For this review, take the finished solid that the model builds, in its own axes (mm). A direction names the side the tool comes from. Coordinates: 2 decimals unless noted, no trailing zeros. Loops run counter-clockwise (first coordinate to the right, second up) from the corner with the lowest first, then second, coordinate; pieces in that order, holes last. Notation, with made-up numbers: M 30,21 L 85,21 A31 cw 85,53 Z; hole C -7.5,-29 d6. An arc over 180 degrees is marked long. Use one line per item in the form item = value.
```python
from build123d import *

# Parameters (mm, degrees)
SKETCH1_W               = 32
SKETCH1_H               = 128
BOSS_EXTRUDE1_DEPTH     = 4
SKETCH4_R               = 1.25
CUT_EXTRUDE2_DEPTH      = 10
SKETCH5_R               = 1.25
CUT_EXTRUDE3_DEPTH      = 10
CUT_EXTRUDE4_DEPTH      = 1.65
LPATTERN3_COUNT         = 4
LPATTERN3_PITCH         = 32
CUT_EXTRUDE5_DEPTH      = 1.65
LPATTERN4_COUNT         = 4
LPATTERN4_PITCH         = 32
SKETCH8_W               = 24.3
SKETCH8_H               = 24.3
CUT_EXTRUDE6_DEPTH      = 10
BOSS_EXTRUDE2_DEPTH     = 4.5
SKETCH11_W              = 10.2
SKETCH11_H              = 71.7
CUT_EXTRUDE7_DEPTH      = 72.92530848
CUT_EXTRUDE8_DEPTH      = 3
SKETCH12_R              = 2.25
CUT_EXTRUDE9_DEPTH      = 3
MIRROR3_COPY_1_DEPTH    = 3
MIRROR3_COPY_2_SKETCH_R = 2.25
MIRROR3_COPY_2_DEPTH    = 3
SKETCH14_W              = 22
SKETCH14_H              = 3.85
CUT_EXTRUDE13_DEPTH     = 10


with BuildPart() as part:
    # Sketch1 → Boss-Extrude1 (new body)
    with BuildSketch(Plane(origin=(0, 0, 0), x_dir=(1, 0, 0), z_dir=(0, 1, 0))):
        Rectangle(SKETCH1_W, SKETCH1_H)
    extrude(amount=BOSS_EXTRUDE1_DEPTH)

    # Sketch4 → Cut-Extrude2 (cut)
    with BuildSketch(Plane.XZ):
        with Locations(Location((13.4, 61.4, 0), (0, 0, 270))):
            Circle(SKETCH4_R)
    cut_extrude2 = extrude(amount=-CUT_EXTRUDE2_DEPTH, mode=Mode.SUBTRACT)

    # Sketch5 → Cut-Extrude3 (cut)
    with BuildSketch(Plane.XZ):
        with Locations(Location((-13.4, -61.4, 0), (0, 0, 270))):
            Circle(SKETCH5_R)
    cut_extrude3 = extrude(amount=-CUT_EXTRUDE3_DEPTH, mode=Mode.SUBTRACT)

    # Sketch6 → Cut-Extrude4 (cut)
    with BuildSketch(Plane(origin=(0, 4, 0), x_dir=(1, 0, 0), z_dir=(0, 1, 0))):
        Polygon((-15.400518683, 62.555), (-13.4, 63.71), (-11.399481317, 62.555), (-11.399481317, 60.245), (-13.4, 59.09), (-15.400518683, 60.245), align=None)
    cut_extrude4 = extrude(amount=-CUT_EXTRUDE4_DEPTH, mode=Mode.SUBTRACT)

    # LPattern3: Cut-Extrude3, Cut-Extrude4 ×4
    with Locations(*[(0, 0, i * LPATTERN3_PITCH) for i in range(1, LPATTERN3_COUNT)]):
        add(cut_extrude3, mode=Mode.SUBTRACT)
        add(cut_extrude4, mode=Mode.SUBTRACT)

    # Sketch7 → Cut-Extrude5 (cut)
    with BuildSketch(Plane(origin=(0, 4, 0), x_dir=(1, 0, 0), z_dir=(0, 1, 0))):
        Polygon((13.4, -59.09), (11.399481317, -60.245), (11.399481317, -62.555), (13.4, -63.71), (15.400518683, -62.555), (15.400518683, -60.245), align=None)
    cut_extrude5 = extrude(amount=-CUT_EXTRUDE5_DEPTH, mode=Mode.SUBTRACT)

    # LPattern4: Cut-Extrude2, Cut-Extrude5 ×4
    with Locations(*[(0, 0, -i * LPATTERN4_PITCH) for i in range(1, LPATTERN4_COUNT)]):
        add(cut_extrude2, mode=Mode.SUBTRACT)
        add(cut_extrude5, mode=Mode.SUBTRACT)

    # Sketch8 → Cut-Extrude6 (cut)
    with BuildSketch(Plane.XZ):
        with Locations((0, 48)):
            Rectangle(SKETCH8_W, SKETCH8_H)
    cut_extrude6 = extrude(amount=-CUT_EXTRUDE6_DEPTH, mode=Mode.SUBTRACT)

    # Mirror1: Cut-Extrude6 across plane
    add(cut_extrude6.mirror(Plane.XY), mode=Mode.SUBTRACT)

    # Sketch9 → Boss-Extrude2 (add)
    with BuildSketch(Plane(origin=(0, 0, -64), x_dir=(-1, 0, 0), z_dir=(0, 0, -1))):
        Polygon((-16, 12), (-5, 12), (-5, 15), (5, 15), (5, 12), (16, 12), (16, -8), (5, -8), (5, -11), (-5, -11), (-5, -8), (-16, -8), align=None)
    boss_extrude2 = extrude(amount=BOSS_EXTRUDE2_DEPTH)

    # Sketch11 → Cut-Extrude7 (cut, through all)
    with BuildSketch(Plane.XZ):
        Rectangle(SKETCH11_W, SKETCH11_H)
    extrude(amount=-CUT_EXTRUDE7_DEPTH, mode=Mode.SUBTRACT)

    # Sketch10 → Cut-Extrude8 (cut)
    with BuildSketch(Plane.XY.offset(-64)):
        Polygon((-2.52, 13.864768035), (2.52, 13.864768035), (5.04, 9.5), (2.52, 5.135231965), (-2.52, 5.135231965), (-5.04, 9.5), align=None)
    cut_extrude8 = extrude(amount=-CUT_EXTRUDE8_DEPTH, mode=Mode.SUBTRACT)

    # Sketch12 → Cut-Extrude9 (cut)
    with BuildSketch(Plane.XY.offset(-67)):
        with Locations((0, 9.5)):
            Circle(SKETCH12_R)
    cut_extrude9 = extrude(amount=-CUT_EXTRUDE9_DEPTH, mode=Mode.SUBTRACT)

    # Mirror2: Cut-Extrude8, Cut-Extrude9 across plane
    add(cut_extrude8.mirror(Plane.ZX.offset(2)), mode=Mode.SUBTRACT)
    add(cut_extrude9.mirror(Plane.ZX.offset(2)), mode=Mode.SUBTRACT)

    # Mirror3: Boss-Extrude2, Cut-Extrude8, Cut-Extrude9 across plane
    add(boss_extrude2.mirror(Plane.XY))
    add(cut_extrude8.mirror(Plane.XY), mode=Mode.SUBTRACT)
    add(cut_extrude9.mirror(Plane.XY), mode=Mode.SUBTRACT)

    # Mirror3 copy 1 sketch → Mirror3 copy 1 (cut)
    with BuildSketch(Plane(origin=(0, 4, 64), x_dir=(1, 0, 0), z_dir=(0, 0, -1))):
        Polygon((-2.52, 13.864768035), (2.52, 13.864768035), (5.04, 9.5), (2.52, 5.135231965), (-2.52, 5.135231965), (-5.04, 9.5), align=None)
    extrude(amount=-MIRROR3_COPY_1_DEPTH, mode=Mode.SUBTRACT)

    # Mirror3 copy 2 sketch → Mirror3 copy 2 (cut)
    with BuildSketch(Plane(origin=(0, 4, 67), x_dir=(1, 0, 0), z_dir=(0, 0, -1))):
        with Locations((0, 9.5)):
            Circle(MIRROR3_COPY_2_SKETCH_R)
    extrude(amount=-MIRROR3_COPY_2_DEPTH, mode=Mode.SUBTRACT)

    # Sketch14 → Cut-Extrude13 (cut)
    with BuildSketch(Plane.XZ):
        with Locations((0, 62.075)):
            Rectangle(SKETCH14_W, SKETCH14_H)
    cut_extrude13 = extrude(amount=-CUT_EXTRUDE13_DEPTH, mode=Mode.SUBTRACT)

    # Mirror4: Cut-Extrude13 across plane
    add(cut_extrude13.mirror(Plane.XY), mode=Mode.SUBTRACT)


solid = part.part
```
1. Consider section C-C on z = -24. Write out the cut boundary in (x, y), plus the area to 3 significant figures.
Computed values:
outline = M -16,0 L -5.1,0 L -5.1,4 L -16,4 Z; M 5.1,0 L 16,0 L 16,4 L 5.1,4 Z
area = 87.2 mm2
2. Consider section D-D on x = 0. State how many separate pieces and enclosed holes the cut face has, plus the area to 3 significant figures.
Computed values:
separate_pieces = 6
enclosed_holes = 0
area = 102 mm2
3. Draft analysis for pull direction X (two halves, no side actions). For faces 1 (the face through (10, -8, 66)), 2 (the face through (-14, 2.35, 4)), 3 (the face through (-5, 14, 66)), state which applies: +X half, -X half, draft (parallel to the pull), parting line (faces both ways), or undercut.
Computed values:
face_1 = draft
face_2 = undercut
face_3 = -X half
4. Consider section B-B on z = -61.4. Write out the cut boundary in (x, y), plus the area to 3 significant figures.
Computed values:
outline = M -16,0 L -14.65,0 L -14.65,2.35 L -15.4,2.35 L -15.4,4 L -16,4 Z; M -12.15,0 L -11,0 L -11,4 L -11.4,4 L -11.4,2.35 L -12.15,2.35 Z; M 11,0 L 16,0 L 16,4 L 11,4 Z
area = 27.5 mm2
5. Consider section A-A on x = 8.5. Write out the cut boundary in (y, z).
Computed values:
outline = M -8,-68.5 L 12,-68.5 L 12,-64 L -8,-64 Z; M -8,64 L 12,64 L 12,68.5 L -8,68.5 Z; M 0,-35.85 L 4,-35.85 L 4,35.85 L 0,35.85 Z
6. Tool access review of faces 4 (the face through (12, 2.35, -2)), 5 (the face through (9, 2, -35.85)), 6 (the face through (-11, -8, 66)), 7 (the face through (-1, 12, -67)), 8 (the face through (11, 12, -66)): name each direction out of +Z, -Z, +X, -X, +Y, -Y from which nothing blocks a thin tool from reaching the whole face with its end or side.
Computed values:
face_4 = +Y
face_5 = +Y, -Y
face_6 = +Z, -Z, -X, -Y
face_7 = none
face_8 = +Z, -Z, +X, +Y
7. Wall thickness on line 1 along X through (y, z) = (0.5, 29.4); line 2 along X through (y, z) = (1.25, -29.4); line 3 along Z through (x, y) = (-13, 5): over which ranges is each line inside the solid? List them lowest first. Write a range as from..to.
Computed values:
line_1 = -16..-5.1, 5.1..12.15, 14.65..16
line_2 = -16..-14.65, -12.15..-5.1, 5.1..16
line_3 = -68.5..-64, 64..68.5
8. For pin 1 Ø5 at (x, z) = (-11, -66.5) entering from +Y; pin 2 Ø2 at (x, z) = (-13.4, -61.4) entering from -Y; pin 3 Ø0.9 at (y, z) = (-9.5, -65.5) entering from +X; pin 4 Ø4 at (x, z) = (-12, -30) entering from -Y, all flat-tipped, find the tip position at first contact; note any pin that passes through.
Computed values:
pin_1 = 12
pin_2 = through
pin_3 = 5
pin_4 = 0
